The model under review builds one solid part; all positions refer to its coordinate system, in mm. A direction names the side the tool comes from. Coordinates: 2 decimals unless noted, no trailing zeros. Order: outer loops, then holes, each group sorted by start corner. A loop starts at its lowest first (then second) coordinate and runs counter-clockwise, first axis right, second up. Notation, with made-up numbers: (23.25, 53.25) -> (61.25, 53.25) arc R32 ccw to (61.25, 79.25) -> close; hole circle Ø3 at (63.25, 74.5). An arc over 180 degrees is marked (long way). Use one line per item in the form item = value. Start each with the question number.
(1) Take a section at A-A (x = 6). State the section outline as (y, z) points (1 decimal).
(2) For faces 1 (the flat face through (-2, 21, -12.5)), 2 (the cylindrical face through (4.9, -1.6, 5)), 3 (the flat face through (-2, 21, -15.675)), list the 3-axis set-ups (+Z, -Z, +X, -X, +Y, -Y) from which the entire face can be reached by the end or side of a thin tool; tool diameter is ignored.
(3) Mouldability with a two-part tool opening along X and no side actions: class faces 4 (the flat face through (7, 17, -14)), 5 (the cylindrical face through (-3.905, -1.565, -0.867)), 6 (the flat face through (5, 41.888, -45)) as +X half, -X half, draft (parallel to the pull), parting line (faces both ways), or undercut.
(4) Take a section at B-B (y = 17). State the section outline as (x, z) points (3 decimals), then the cut area to 4 significant figures.
(5) Wall thickness on line 1 along Z through (x, y) = (1.5, 17.5) (3 decimals); line 2 along Y through (x, z) = (10.5, -60); line 3 along Y through (x, z) = (-9, -4) (3 decimals): over which ranges is each line inside the solid? List them lowest first.
(6) Insertion check: pin 1 Ø3 at (x, y) = (-5.5, 26.5) entering from +Z; pin 2 Ø5 at (x, y) = (1.5, 13) entering from -Z (3 decimals); pin 3 Ø13 at (x, z) = (0, 0) entering from +Y. Each pin has a flat end and moves straight along its axis. Give the tip position at first contact, or say it passes through.
(7) Take a section at C-C (z = -42.5). State the section outline as (x, y) points, then the cut area to 3 significant figures.
```python
from build123d import *

# Parameters (mm, degrees)
SKETCH1_R                    = 4
BASE_FLANGE1_DEPTH           = 3.175
EDGE_FLANGE1_STRIP_W         = 14.1732
EDGE_FLANGE1_STRIP_H         = 3.175
EDGE_FLANGE1_STRIP_CUT_DEPTH = 18
EDGE_FLANGE1_DEPTH           = 18
EDGE_FLANGE2_STRIP_W         = 14.1732
EDGE_FLANGE2_STRIP_H         = 3.175
EDGE_FLANGE2_STRIP_CUT_DEPTH = 18
EDGE_FLANGE2_DEPTH           = 18
SKETCH12_R                   = 4.125
BOSS_EXTRUDE1_DEPTH          = 3.175


# Sheet-metal steps are written as plain solids
with BuildPart() as part:
    # Sketch1 → Base-Flange1 (new body)
    with BuildSketch(Plane(origin=(0, 0, 0), x_dir=(1, 0, 0), z_dir=(0, 1, 0))):
        with BuildLine():
            Line((7, 0), (7, 12.5))
            Line((7, 12.5), (-11, 12.5))
            Line((-11, 12.5), (-11, 0))
            ThreePointArc((-11, 0), (-8.949747468, -4.949747468), (-4, -7))
            Line((-4, -7), (0, -7))
            ThreePointArc((0, -7), (4.949747468, -4.949747468), (7, 0))
        make_face()
        with Locations(Location((0, 0, 0), (0, 0, 270))):
            Circle(SKETCH1_R, mode=Mode.SUBTRACT)
    extrude(amount=-BASE_FLANGE1_DEPTH)

    # Edge-Flange1 strip (across the edge) → Edge-Flange1 strip cut (cut)
    with BuildSketch(Plane(origin=(7, 0, -12.5), x_dir=(0, 0, 1), z_dir=(-1, 0, 0))):
        with Locations((-6.35, -1.5875)):
            Rectangle(EDGE_FLANGE1_STRIP_W, EDGE_FLANGE1_STRIP_H)
    extrude(amount=EDGE_FLANGE1_STRIP_CUT_DEPTH, mode=Mode.SUBTRACT)

    # Edge-Flange1 section (across the edge) → Edge-Flange1 (add)
    with BuildSketch(Plane(origin=(7, 0, -12.5), x_dir=(0, 0, 1), z_dir=(-1, 0, 0))):
        with BuildLine():
            Line((-3.175, 0.7366), (-3.175, 41.8875))
            Line((-3.175, 41.8875), (0, 41.8875))
            Line((0, 41.8875), (0, 0.7366))
            ThreePointArc((0, 0.7366), (0.215745145, 0.215745145), (0.7366, 0))
            Line((0.7366, 0), (0.7366, -3.175))
            ThreePointArc((0.7366, -3.175), (-2.029318885, -2.029318885), (-3.175, 0.7366))
        make_face()
    extrude(amount=EDGE_FLANGE1_DEPTH)

    # Edge-Flange2 strip (across the edge) → Edge-Flange2 strip cut (cut)
    with BuildSketch(Plane(origin=(-11, 41.8875, -15.675), x_dir=(0, -1, 0), z_dir=(1, 0, 0))):
        with Locations((-6.35, -1.5875)):
            Rectangle(EDGE_FLANGE2_STRIP_W, EDGE_FLANGE2_STRIP_H)
    extrude(amount=EDGE_FLANGE2_STRIP_CUT_DEPTH, mode=Mode.SUBTRACT)

    # Edge-Flange2 section (across the edge) → Edge-Flange2 (add)
    with BuildSketch(Plane(origin=(-11, 41.8875, -15.675), x_dir=(0, -1, 0), z_dir=(1, 0, 0))):
        with BuildLine():
            Line((-3.175, 0.7366), (-3.175, 3))
            Line((-3.175, 3), (0, 3))
            Line((0, 3), (0, 0.7366))
            ThreePointArc((0, 0.7366), (0.215745145, 0.215745145), (0.7366, 0))
            Line((0.7366, 0), (0.7366, -3.175))
            ThreePointArc((0.7366, -3.175), (-2.029318885, -2.029318885), (-3.175, 0.7366))
        make_face()
    extrude(amount=EDGE_FLANGE2_DEPTH)

    # Sketch12 → Boss-Extrude1 (add)
    with BuildSketch(Plane(origin=(0, 45.0625, 0), x_dir=(1, 0, 0), z_dir=(0, 1, 0))):
        with BuildLine():
            Line((7, 18.675), (-11, 18.675))
            ThreePointArc((-11, 18.675), (-10.657865377, 23.027974643), (-9.639863923, 27.27404546))
            Line((-9.639863923, 27.27404546), (3.238154817, 66.964241218))
            ThreePointArc((3.238154817, 66.964241218), (7.212761051, 71.621798227), (13.316622217, 72.104717351))
            Line((13.316622217, 72.104717351), (15.218990158, 71.487468443))
            ThreePointArc((15.218990158, 71.487468443), (19.876547167, 67.512862208), (20.359466291, 61.409001043))
            Line((20.359466291, 61.409001043), (7.481447551, 21.718805285))
            ThreePointArc((7.481447551, 21.718805285), (7.121105439, 20.215823024), (7, 18.675))
        make_face()
        with Locations(Location((12.749994525, 63.877996676, 0), (0, 0, 270))):
            Circle(SKETCH12_R, mode=Mode.SUBTRACT)
    extrude(amount=-BOSS_EXTRUDE1_DEPTH)


solid = part.part
```
Findings:
q1.outline = (-3.2, -11.8) arc R3.9 ccw to (0.7, -15.7) -> (41.2, -15.7) arc R0.7 cw to (41.9, -16.4) -> (41.9, -70.9) -> (45.1, -70.9) -> (45.1, -16.4) arc R3.9 ccw to (41.2, -12.5) -> (0.7, -12.5) arc R0.7 cw to (0, -11.8) -> (0, 3.6) -> (-3.2, 3.6) -> close
q2.face_1 = +Z, +X, -X, +Y
q2.face_2 = +Z, +X, +Y, -Y
q2.face_3 = -Z, +X, -X, -Y
q3.face_4 = +X half
q3.face_5 = undercut
q3.face_6 = draft
q4.outline = (-11, -15.675) -> (7, -15.675) -> (7, -12.5) -> (-11, -12.5) -> close
q4.area = 57.15 mm²
q5.line_1 = -15.675 to -12.5
q5.line_2 = 41.89 to 45.06
q5.line_3 = -3.175 to 0
q6.pin_1 = -12.5
q6.pin_2 = -15.675
q6.pin_3 = 0
q7.outline = (-4.7, 41.89) -> (14.22, 41.89) -> (14.22, 45.06) -> (-4.7, 45.06) -> close
q7.area = 60.1 mm²
